```python
from build123d import *

# Parameters (mm, degrees)
BOSS_EXTRUDE1_DEPTH                          = 27.5
CBORE_FOR_M6_HEX_SOCKET_HEAD_CAP_SCR_2_COUNT = 2
CBORE_FOR_M6_HEX_SOCKET_HEAD_CAP_SCR_2_PITCH = 33
CBORE_FOR_M6_HEX_SOCKET_HEAD_CAP_SCR_3_COUNT = 2
CBORE_FOR_M6_HEX_SOCKET_HEAD_CAP_SCR_3_PITCH = 46.669047558
CBORE_FOR_M6_HEX_SOCKET_HEAD_CAP_SCR_4_COUNT = 2
CBORE_FOR_M6_HEX_SOCKET_HEAD_CAP_SCR_4_PITCH = 33
SKETCH8_R                                    = 15
CUT_EXTRUDE3_DEPTH                           = 10
SKETCH9_W                                    = 1
SKETCH9_H                                    = 7.727187909
SKETCH9_W_2                                  = 7.727187909
SKETCH9_H_2                                  = 1
EXTRUDE_THIN3_DEPTH                          = 5
FILLET1_R                                    = 1
SKETCH10_R                                   = 14
BOSS_EXTRUDE2_DEPTH                          = 15
FILLET2_R                                    = 1
SKETCH11_R                                   = 6
CUT_EXTRUDE4_DEPTH                           = 54.091901454
SKETCH12_R                                   = 16
SKETCH12_R_2                                 = 6
BOSS_EXTRUDE3_DEPTH                          = 5
SKETCH14_R                                   = 3.175
CUT_EXTRUDE6_DEPTH                           = 10
CHAMFER2_SIZE                                = 0.5


with BuildPart() as part:
    # Sketch1 → Boss-Extrude1 (new body)
    with BuildSketch(Plane(origin=(0, 0, 0), x_dir=(1, 0, 0), z_dir=(0, 1, 0))):
        with BuildLine():
            Line((-19.5, -22.5), (19.5, -22.5))
            ThreePointArc((19.5, -22.5), (21.621320344, -21.621320344), (22.5, -19.5))
            Line((22.5, -19.5), (22.5, 19.5))
            ThreePointArc((22.5, 19.5), (21.621320344, 21.621320344), (19.5, 22.5))
            Line((19.5, 22.5), (-19.5, 22.5))
            ThreePointArc((-19.5, 22.5), (-21.621320344, 21.621320344), (-22.5, 19.5))
            Line((-22.5, 19.5), (-22.5, -19.5))
            ThreePointArc((-22.5, -19.5), (-21.621320344, -21.621320344), (-19.5, -22.5))
        make_face()
    extrude(amount=BOSS_EXTRUDE1_DEPTH)

    # Sketch3 → CBORE for M6 Hex Socket Head Cap Screw1 (revolve, cut)
    with BuildSketch(Plane(origin=(-16.5, 27.5, -16.5), x_dir=(0, 0, 1), z_dir=(1, 0, 0))):
        Polygon((0, 0), (0, 27.5), (3.2, 27.5), (3.2, 15), (4.75, 15), (4.75, 0.25), (5, 0), align=None)
    cbore_for_m6_hex_socket_head_cap_screw1 = revolve(axis=Axis((-16.5, 33.85, -16.5), (0, -1, 0)), mode=Mode.SUBTRACT)

    # CBORE for M6 Hex Socket Head Cap Scr 2: CBORE for M6 Hex Socket Head Cap Screw1 ×2
    with Locations(*[(i * CBORE_FOR_M6_HEX_SOCKET_HEAD_CAP_SCR_2_PITCH, 0, 0) for i in range(1, CBORE_FOR_M6_HEX_SOCKET_HEAD_CAP_SCR_2_COUNT)]):
        add(cbore_for_m6_hex_socket_head_cap_screw1, mode=Mode.SUBTRACT)

    # CBORE for M6 Hex Socket Head Cap Scr 3: CBORE for M6 Hex Socket Head Cap Screw1 ×2
    with Locations(*[Vector(0.7071067811865476, 0, 0.7071067811865475) * (i * CBORE_FOR_M6_HEX_SOCKET_HEAD_CAP_SCR_3_PITCH) for i in range(1, CBORE_FOR_M6_HEX_SOCKET_HEAD_CAP_SCR_3_COUNT)]):
        add(cbore_for_m6_hex_socket_head_cap_screw1, mode=Mode.SUBTRACT)

    # CBORE for M6 Hex Socket Head Cap Scr 4: CBORE for M6 Hex Socket Head Cap Screw1 ×2
    with Locations(*[(0, 0, i * CBORE_FOR_M6_HEX_SOCKET_HEAD_CAP_SCR_4_PITCH) for i in range(1, CBORE_FOR_M6_HEX_SOCKET_HEAD_CAP_SCR_4_COUNT)]):
        add(cbore_for_m6_hex_socket_head_cap_screw1, mode=Mode.SUBTRACT)

    # Sketch8 → Cut-Extrude3 (cut)
    with BuildSketch(Plane(origin=(0, 27.5, 0), x_dir=(1, 0, 0), z_dir=(0, 1, 0))):
        with BuildLine():
            ThreePointArc((-9.5, -16.5), (-11.550252532, -11.550252532), (-16.5, -9.5))
            Line((-16.5, -9.5), (-20.5, -9.5))
            Line((-20.5, -9.5), (-20.5, 0))
            Line((-20.5, 0), (-20.5, 9.5))
            Line((-20.5, 9.5), (-16.5, 9.5))
            ThreePointArc((-16.5, 9.5), (-11.550252532, 11.550252532), (-9.5, 16.5))
            Line((-9.5, 16.5), (-9.5, 20.5))
            Line((-9.5, 20.5), (0, 20.5))
            Line((0, 20.5), (9.5, 20.5))
            Line((9.5, 20.5), (9.5, 16.5))
            ThreePointArc((9.5, 16.5), (11.550252532, 11.550252532), (16.5, 9.5))
            Line((16.5, 9.5), (20.5, 9.5))
            Line((20.5, 9.5), (20.5, 0))
            Line((20.5, 0), (20.5, -9.5))
            Line((20.5, -9.5), (16.5, -9.5))
            ThreePointArc((16.5, -9.5), (11.550252532, -11.550252532), (9.5, -16.5))
            Line((9.5, -16.5), (9.5, -20.5))
            Line((9.5, -20.5), (0, -20.5))
            Line((0, -20.5), (-9.5, -20.5))
            Line((-9.5, -20.5), (-9.5, -16.5))
        make_face()
        with Locations(Location((0, 0, 0), (0, 0, 270))):
            Circle(SKETCH8_R, mode=Mode.SUBTRACT)
    extrude(amount=-CUT_EXTRUDE3_DEPTH, mode=Mode.SUBTRACT)

    # Sketch9 → Extrude-Thin3 (add)
    with BuildSketch(Plane(origin=(0, 17.5, 0), x_dir=(1, 0, 0), z_dir=(0, 1, 0))):
        with Locations((0, 17.395249071)):
            Rectangle(SKETCH9_W, SKETCH9_H)
        Polygon((-9.522770805, 10.229877587), (-11.660876198, 12.367982979), (-12.367982979, 11.660876198), (-10.229877587, 9.522770805), align=None)
        with Locations((17.395249071, 0)):
            Rectangle(SKETCH9_W_2, SKETCH9_H_2)
        Polygon((10.229877587, 9.522770805), (12.367982979, 11.660876198), (11.660876198, 12.367982979), (9.522770805, 10.229877587), align=None)
        with Locations((0, -17.395249071)):
            Rectangle(SKETCH9_W, SKETCH9_H)
        Polygon((9.522770805, -10.229877587), (11.660876198, -12.367982979), (12.367982979, -11.660876198), (10.229877587, -9.522770805), align=None)
        with Locations((-17.395249071, 0)):
            Rectangle(SKETCH9_W_2, SKETCH9_H_2)
        Polygon((-10.229877587, -9.522770805), (-12.367982979, -11.660876198), (-11.660876198, -12.367982979), (-9.522770805, -10.229877587), align=None)
    extrude(amount=EXTRUDE_THIN3_DEPTH)

    # Fillet1
    fillet1_edges = [part.edges().sort_by_distance(p)[0] for p in [
        (-20.5, 22.5, 9.5),
        (-20.5, 22.5, -9.5),
        (-9.5, 22.5, -20.5),
        (9.5, 22.5, -20.5),
        (20.5, 22.5, -9.5),
        (20.5, 22.5, 9.5),
        (9.5, 22.5, 20.5),
        (-9.5, 22.5, 20.5),
    ]]
    fillet(fillet1_edges, radius=FILLET1_R)

    # Sketch10 → Boss-Extrude2 (add)
    with BuildSketch(Plane(origin=(0, 27.5, 0), x_dir=(1, 0, 0), z_dir=(0, 1, 0))):
        with Locations(Location((0, 0, 0), (0, 0, 270))):
            Circle(SKETCH10_R)
    extrude(amount=BOSS_EXTRUDE2_DEPTH)

    # Fillet2
    fillet2_edges = [part.edges().sort_by_distance(p)[0] for p in [
        (0, 42.5, -14),
    ]]
    fillet(fillet2_edges, radius=FILLET2_R)

    # Sketch11 → Cut-Extrude4 (cut, through all)
    with BuildSketch(Plane(origin=(0, 42.5, 0), x_dir=(1, 0, 0), z_dir=(0, 1, 0))):
        with Locations(Location((0, 0, 0), (0, 0, 270))):
            Circle(SKETCH11_R)
    extrude(amount=-CUT_EXTRUDE4_DEPTH, mode=Mode.SUBTRACT)

    # Sketch12 → Boss-Extrude3 (add)
    with BuildSketch(Plane.XZ):
        with Locations(Location((0, 0, 0), (0, 0, 270))):
            Circle(SKETCH12_R)
        with Locations(Location((0, 0, 0), (0, 0, 90))):
            Circle(SKETCH12_R_2, mode=Mode.SUBTRACT)
    extrude(amount=BOSS_EXTRUDE3_DEPTH)

    # Sketch14 → Cut-Extrude6 (cut)
    with BuildSketch(Plane(origin=(0, 0, -22.5), x_dir=(-1, 0, 0), z_dir=(0, 0, -1))):
        with Locations((-5.5, 13.75)):
            Circle(SKETCH14_R)
    extrude(amount=-CUT_EXTRUDE6_DEPTH, mode=Mode.SUBTRACT)

    # Chamfer2
    chamfer2_edges = [part.edges().sort_by_distance(p)[0] for p in [
        (8.675, 13.75, -22.5),
    ]]
    chamfer(chamfer2_edges, length=CHAMFER2_SIZE)


solid = part.part
```
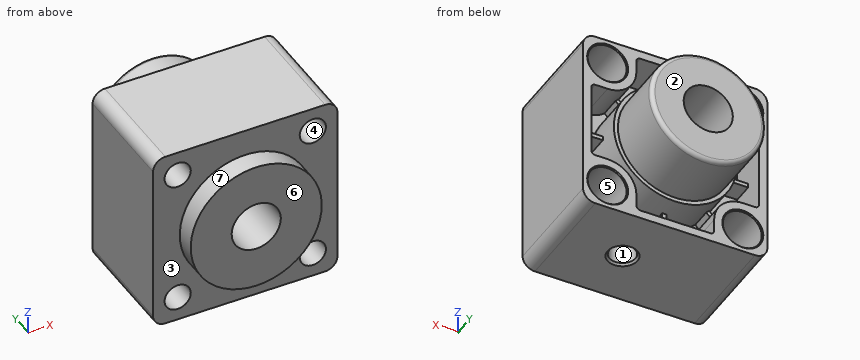
Part model, mm, in its own coordinate system. Face numbers are marked on the shaded views. A direction names the side the tool comes from. Coordinates: 2 decimals unless noted, no trailing zeros. Write each loop counter-clockwise with the first axis right and the second up, starting at its lowest first coordinate (ties: lowest second). Pieces come first, ordered by that corner, then holes.
Item 1: Mould opens along Y. For the marked faces 1, 2, 3 and 4 say: released by +Y, released by -Y, zero draft, split by the parting line, or undercut.
Item 2: Slice it at B-B (y = 26.5). Count the separate pieces of the cut face and the enclosed holes in it, and give its area (3 significant figures).
Item 3: Probe line 1 (X direction, y = 21.5, z = -16.5); line 2 (Z direction, x = 16.5, y = 16.75). List the from-to ranges inside material, lowest first.
Item 4: Which spindle directions (+Z, -Z, +X, -X, +Y, -Y) get a long thin tool onto all of the face, cutting with end or side? Do the marked faces 5, 6 and 7. Say none if no direction does.
Item 5: Slice it at A-A (y = 13.75). Write the cut outline in (x, z) (3 decimals).
Item 6: Pin check, flat tips, straight feed: pin 1 (0.5 mm diameter, centred on x = 18, z = 0, fed in from +Y); pin 2 (5 mm diameter, centred on x = 7, z = -14.5, fed in from +Y); pin 3 (2 mm diameter, centred on x = 5.5, z = -17, fed in from +Y). Stop position of each tip, or through.
Results found:
1. face 1: undercut
1. face 2: released by +Y
1. face 3: released by -Y
1. face 4: zero draft
2. separate pieces: 2
2. enclosed holes: 6
2. area: 1,090 mm2
3. line 1: x = -22.5 to -21.25, -11.75 to -9.5, -0.5 to 0.5, 9.5 to 11.75, 21.25 to 22.5
3. line 2: z = -22.5 to -21.25, -11.75 to 11.75, 21.25 to 22.5
4. face 5: +Y
4. face 6: +Z, -Z, +X, -X, -Y
4. face 7: -Y
5. outline: (-22.5, -19.5) arc R3 ccw to (-19.5, -22.5) - (1.825, -22.5) - (2.325, -22) - (2.325, -12.5) - (8.675, -12.5) - (8.675, -22) - (9.175, -22.5) - (19.5, -22.5) arc R3 ccw to (22.5, -19.5) - (22.5, 19.5) arc R3 ccw to (19.5, 22.5) - (-19.5, 22.5) arc R3 ccw to (-22.5, 19.5) - close; hole circle Ø9.5 at (-16.5, -16.5); hole circle Ø9.5 at (-16.5, 16.5); hole circle Ø12 at (0, 0); hole circle Ø9.5 at (16.5, -16.5); hole circle Ø9.5 at (16.5, 16.5)
6. pin 1: stops at y = 22.5
6. pin 2: stops at y = 42.3
6. pin 3: stops at y = 17.5
